Could you check a few things on this drawing? It's one solid part, dimensions in mm from its lowest x, y, z. Give positions to 0.01 mm unless a question says otherwise; leave off trailing zeros. Loops run counter-clockwise (first coordinate to the right, second up) from the corner with the lowest first, then second, coordinate; pieces in that order, holes last. Notation, with made-up numbers: M -7,16 L 7,16 A15 ccw 7,34 Z; hole C 72.5,39 d9. An arc over 180 degrees is marked long. Return JSON: item names as keys, results as strings. Group by question number.
1. If we section it at C-C (x = 484): Write out the boundary of the cut face in (y, z), plus the area to 3 significant figures.
2. Please list where these lines run through material, in increasing order: line 1 (Z direction, x = 280, y = 304.5); line 2 (Y direction, x = 161, z = 348); line 3 (Y direction, x = 507, z = 475).
3. If we section it at A-A (z = 300): Write out the boundary of the cut face in (x, y), plus the area to 3 significant figures.
4. For pin 1 (1 mm diameter, centred on x = 277.5, z = 123, fed in from -Y); pin 2 (1 mm diameter, centred on x = 74.5, z = 106.5, fed in from +Y); pin 3 (10 mm diameter, centred on y = 222, z = 217.5, fed in from -X); pin 4 (6 mm diameter, centred on x = 103, y = 374.5, fed in from +Z) (3 decimals), each with a flat end and sliding along its axis, tell me the tip position at first contact or that it passes through.
5. If we section it at B-B (x = 68): Write out the boundary of the cut face in (y, z).
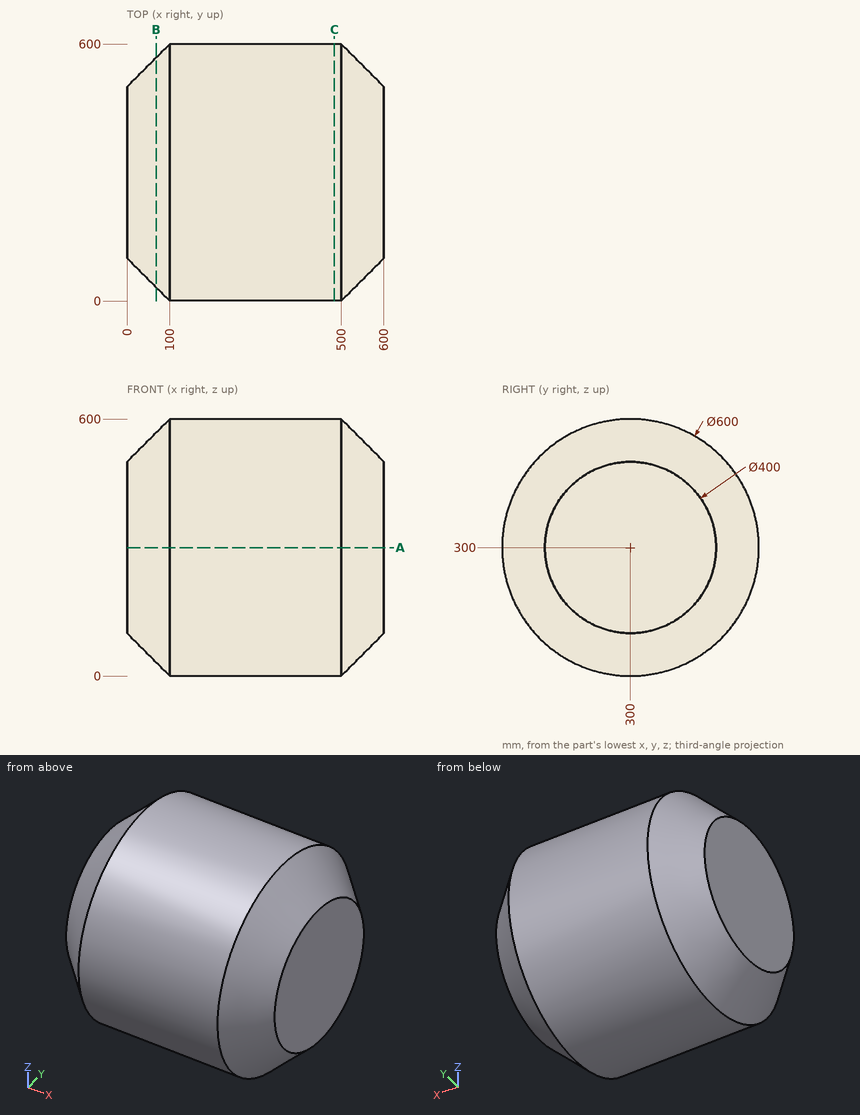
Answer:
{
 "1": {"outline": "C 300,300 d600", "area": "283,000 mm²"},
 "2": {"line 1": "z = 0.03 to 599.97", "line 2": "y = 3.86 to 596.14", "line 3": "y = 65 to 535"},
 "3": {"outline": "M 0,100 L 100,0 L 500,0 L 600,100 L 600,500 L 500,600 L 100,600 L 0,500 Z", "area": "340,000 mm²"},
 "4": {"pin 1": "stops at y = 57.41", "pin 2": "stops at y = 495.56", "pin 3": "stops at x = 0", "pin 4": "stops at z = 591.355"},
 "5": {"outline": "C 300,300 d536"}
}
